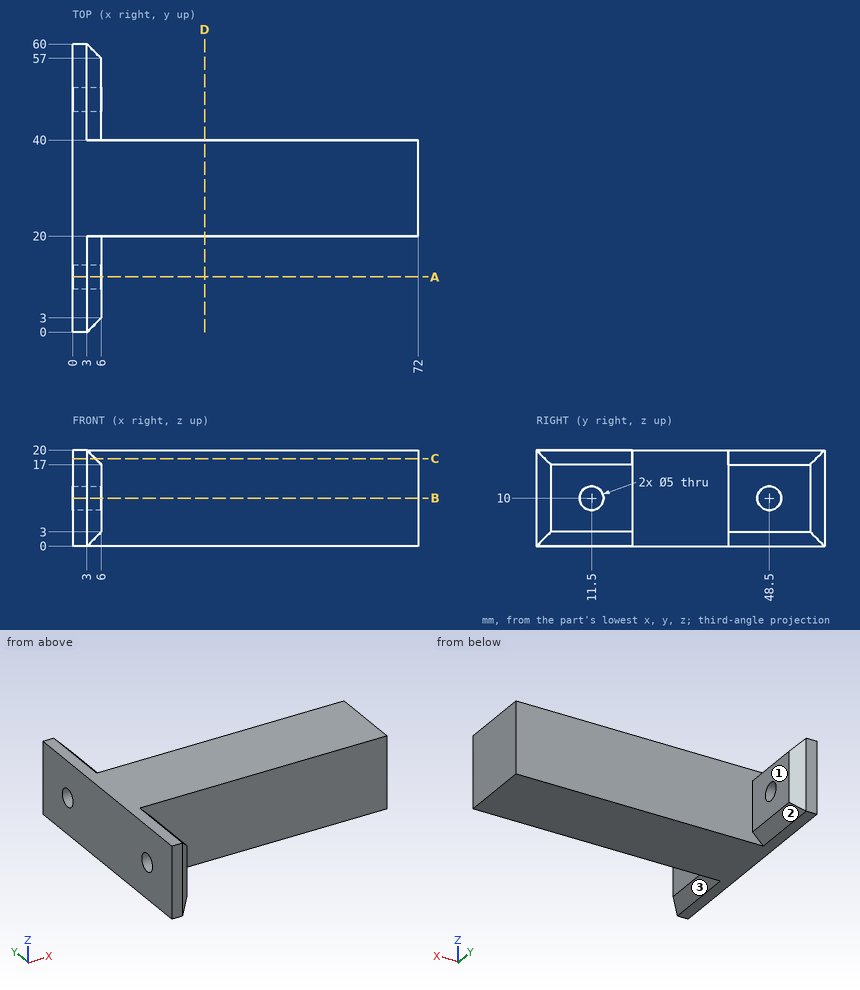
Job drawing, mm, ordinate dimensions from the low corner. One solid piece. A direction names the side the tool comes from. Coordinates: 2 decimals unless noted, no trailing zeros. Write each loop counter-clockwise with the first axis right and the second up, starting at its lowest first coordinate (ties: lowest second). Pieces come first, ordered by that corner, then holes. Notation, with made-up numbers: M 68,16.25 L 93,16.25 A26 cw 93,46.25 Z; hole C -30.75,3 d1. An arc over 180 degrees is marked long. Answer as a JSON object with one key per item and string values. Group by question number.
1) Saw through at C-C (z = 18.25). Write the cut outline in (x, y), plus the area to 3 significant figures.
2) Tool access for the marked faces 1, 2 and 3: list every direction of +Z, -Z, +X, -X, +Y, -Y with a clear straight run to the whole face (end or side of a thin tool).
3) Wall check: line 1 (Y direction, x = 1.55, z = 10); line 2 (Z direction, x = 2.7, y = 48.5); line 3 (Y direction, x = 4.75, z = 10). Give the ranges that are in metal, low to high. Write a range as from..to.
4) Saw through at D-D (x = 27.5). Write the cut outline in (y, z).
5) Saw through at B-B (z = 10). Write the cut outline in (x, y), plus the area to 3 significant figures.
6) Saw through at A-A (y = 11.5). Write the cut outline in (x, z).
7) Pin check, flat tips, straight feed: pin 1 Ø10 at (x, z) = (54.5, 15) entering from +Y; pin 2 Ø4 at (y, z) = (49.5, 7.5) entering from +X; pin 3 Ø4 at (x, z) = (52.5, 6.5) entering from -Y. Stop position of each tip, or through.
Values follow:
{
 "1": {"outline": "M 0,0 L 3,0 L 4.75,1.75 L 4.75,20 L 72,20 L 72,40 L 4.75,40 L 4.75,58.25 L 3,60 L 0,60 Z", "area": "1,630 mm2"},
 "2": {"face 1": "+Z, -Z, +X, +Y", "face 2": "-Z, +X, +Y", "face 3": "-Z, +X, -Y"},
 "3": {"line 1": "y = 0..9, 14..46, 51..60", "line 2": "z = 0..7.5, 12.5..20", "line 3": "y = 1.75..9, 14..46, 51..58.25"},
 "4": {"outline": "M 20,0 L 40,0 L 40,20 L 20,20 Z"},
 "5": {"outline": "M 0,0 L 3,0 L 6,3 L 6,9 L 0,9 Z; M 0,14 L 6,14 L 6,20 L 72,20 L 72,40 L 6,40 L 6,46 L 0,46 Z; M 0,51 L 6,51 L 6,57 L 3,60 L 0,60 Z", "area": "1,610 mm2"},
 "6": {"outline": "M 0,0 L 3,0 L 6,3 L 6,7.5 L 0,7.5 Z; M 0,12.5 L 6,12.5 L 6,17 L 3,20 L 0,20 Z"},
 "7": {"pin 1": "stops at y = 40", "pin 2": "stops at x = 6", "pin 3": "stops at y = 20"}
}
